For this review, take the finished solid that the model builds, in its own axes (mm). A direction names the side the tool comes from. Round coordinates to 2 decimals unless told otherwise and drop trailing zeros. Write each loop counter-clockwise with the first axis right and the second up, starting at its lowest first coordinate (ties: lowest second). Pieces come first, ordered by that corner, then holes. Notation, with made-up numbers: (79, 51) -> (88, 51) arc R23 cw to (88, 77) -> close; hole circle Ø5 at (57.5, 43.5). An arc over 180 degrees is marked (long way). Answer in a Markdown table with one row per item.
Autodesk Inventor part; units mm, degrees
ref_plane "YZ Plane" through (0, 0, 0) normal (1, 0, 0) x (0, 1, 0)
ref_plane "XZ Plane" through (0, 0, 0) normal (0, 1, 0) x (-1, 0, 0)
ref_plane "XY Plane" through (0, 0, 0) normal (0, 0, 1) x (1, 0, 0)
sketch "Sketch3" plane through (0, 0, 0) normal (0, 0, 1) x (1, 0, 0)
  line L0 (0, 0) -> (19.05, 0)
  line L1 (19.05, 0) -> (19.05, -254)
  line L2 (19.05, -254) -> (0, -254)
  line L3 (0, -254) -> (0, 0)
  dimension "d0" = 19.05
  dimension "d1" = 254
extrude "Extrusion1" add sketch "Sketch3" along normal blind 6.35
sketch "Sketch4" plane through (19.05, -254, 0) normal (1, 0, 0) x (0, 0, -1)
  point P0 (0, 254)
sketch "Sketch5" plane through (0, 0, 6.35) normal (0, 0, 1) x (1, 0, 0)
  line L0 (19.05, 0) -> (0, 0)
  line L1 (0, 0) -> (0, -31.75)
  line L2 (0, 0) -> (0, -254)
  line L3 (19.05, -254) -> (19.05, 0)
  line L4 (0, -31.75) -> (19.05, -31.75)
  line L5 (19.05, -31.75) -> (19.05, -38.1)
  line L6 (19.05, -38.1) -> (0, -38.1)
  line L7 (0, -38.1) -> (0, -31.75)
  dimension "d4" = 31.75
  dimension "d5" = 6.35
extrude "Extrusion2" add sketch "Sketch5" along normal blind 88.9 contours L3 L6 L2 L4
sketch "Sketch6" plane through (0, 0, 0) normal (0, 0, -1) x (-1, 0, 0)
  line L0 (-19.05, -31.75) -> (-19.05, 0)
  line L1 (0, 0) -> (-19.05, 0)
  line L2 (-19.05, 0) -> (-19.05, -6.35)
  line L3 (-19.05, -6.35) -> (0, -6.35)
  line L4 (0, -6.35) -> (0, 0)
  dimension "d8" = 6.35
extrude "Extrusion3" add sketch "Sketch6" along normal blind 50.8
fillet "Fillet2" radius 6.35 2 edges at (9.525, -38.1, 6.35) (9.525, -6.35, 0)
sketch "Sketch7" plane through (0, 0, 6.35) normal (0, 0, 1) x (1, 0, 0)
  line L0 (0, -254) -> (19.05, -254)
  line L1 (0, -254) -> (19.05, -254)
  line L2 (19.05, -254) -> (19.05, -247.65)
  line L3 (19.05, -247.65) -> (0, -247.65)
  line L4 (0, -247.65) -> (0, -254)
  point P0 (0, 0)
  dimension "d13" = 19.05
  dimension "d14" = 6.35
extrude "Extrusion4" add sketch "Sketch7" along normal blind 50.8
sketch "Sketch8" plane through (0, 0, 0) normal (0, 0, -1) x (-1, 0, 0)
  line L0 (-19.05, -254) -> (0, -254)
  line L1 (0, -254) -> (0, -12.7)
  line L2 (-19.05, -254) -> (0, -254)
  line L3 (0, -254) -> (0, -247.65)
  line L4 (0, -247.65) -> (-19.05, -247.65)
  line L5 (-19.05, -247.65) -> (-19.05, -254)
  point P0 (0, 0)
  dimension "d17" = 6.35
extrude "Extrusion5" add sketch "Sketch8" along normal blind 50.8
fillet "Fillet3" radius 6.35 2 edges at (9.525, -247.65, 0) (9.525, -247.65, 6.35)
properties part number "RightTopPlateConnector"
1) For line 1 (Y direction, x = 15.75, z = -45); line 2 (Y direction, x = 15.5, z = 33.5); line 3 (Z direction, x = 13, y = -146), list the stretches that pass through material, from the lowest coordinate up. Write a range as [from, to].
Solved:
| item | result |
|---|---|
| line 1 | [-254, -247.65], [-6.35, 0] |
| line 2 | [-254, -247.65], [-38.1, -31.75] |
| line 3 | [0, 6.35] |
2) Consider section A-A on z = 42.5. State the section outline as (x, y) points, then the cut area to 3 significant figures.
Solved:
| item | result |
|---|---|
| outline | (0, -254) -> (19.05, -254) -> (19.05, -247.65) -> (0, -247.65) -> close; (0, -38.1) -> (19.05, -38.1) -> (19.05, -31.75) -> (0, -31.75) -> close |
| area | 242 mm² |
3) Consider section D-D on z = 82. State the section outline as (x, y) points, then the cut area to 3 significant figures.
Solved:
| item | result |
|---|---|
| outline | (0, -38.1) -> (19.05, -38.1) -> (19.05, -31.75) -> (0, -31.75) -> close |
| area | 121 mm² |
4) Consider section B-B on x = 4.5. State the section outline as (y, z) points.
Solved:
| item | result |
|---|---|
| outline | (-254, -50.8) -> (-247.65, -50.8) -> (-247.65, -6.35) arc R6.35 cw to (-241.3, 0) -> (-12.7, 0) arc R6.35 cw to (-6.35, -6.35) -> (-6.35, -50.8) -> (0, -50.8) -> (0, 6.35) -> (-31.75, 6.35) -> (-31.75, 95.25) -> (-38.1, 95.25) -> (-38.1, 12.7) arc R6.35 cw to (-44.45, 6.35) -> (-241.3, 6.35) arc R6.35 cw to (-247.65, 12.7) -> (-247.65, 57.15) -> (-254, 57.15) -> close |
5) For faces 5 (the cylindrical face through (9.39, -39.91, 8.26)), 6 (the flat face through (9, -125, 0)), 7 (the flat face through (9, -16, 6.35)), list the 3-axis set-ups (+Z, -Z, +X, -X, +Y, -Y) from which the entire face can be reached by the end or side of a thin tool; tool diameter is ignored.
Solved:
| item | result |
|---|---|
| face 5 | +Z, +X, -X |
| face 6 | -Z, +X, -X |
| face 7 | +Z, +X, -X, +Y |
6) Clearance check with flat-ended pins moving along their axes: pin 1 Ø3 at (x, y) = (12, -249.5) entering from +Z; pin 2 Ø9.5 at (x, y) = (12, -111) entering from -Z; pin 3 Ø8 at (x, z) = (12.5, 48.5) entering from +Y. State where each tip first meets the part, or that it passes through.
Solved:
| item | result |
|---|---|
| pin 1 | z = 57.15 |
| pin 2 | z = 0 |
| pin 3 | y = -31.75 |
7) Mouldability with a two-part tool opening along Y and no side actions: class faces 1 (the flat face through (10, -254, 4)), 2 (the flat face through (10, -38.1, 53)), 3 (the flat face through (9, 0, -22)), 4 (the flat face through (10, -3, -50.8)) as pulls with the +Y half, pulls with the -Y half, needs draft (parallel to the pull), parting line crosses it, or undercut.
Solved:
| item | result |
|---|---|
| face 1 | pulls with the -Y half |
| face 2 | undercut |
| face 3 | pulls with the +Y half |
| face 4 | needs draft |
8) Consider section C-C on y = -225. State the section outline as (x, z) points, then the cut area to 3 significant figures.
Solved:
| item | result |
|---|---|
| outline | (0, 0) -> (19.05, 0) -> (19.05, 6.35) -> (0, 6.35) -> close |
| area | 121 mm² |
